Build history of the part. All positions in model axes, mm. A direction names the side the tool comes from. Coordinates: 2 decimals unless noted, no trailing zeros. Loops run counter-clockwise (first coordinate to the right, second up) from the corner with the lowest first, then second, coordinate; pieces in that order, holes last.
Item 1: Mould opens along Y. For faces 1 (the face through (2.321, 11.223, 1.479)), 2 (the face through (10, 0, 1)), 3 (the face through (5, 9, 1)) say: released by +Y, released by -Y, zero draft, split by the parting line, or undercut.
Item 2: Flat gauge pins, fed straight in: pin 1 (1.6 mm diameter, centred on x = 17.5, y = 2.5, fed in from -Z); pin 2 (1.5 mm diameter, centred on x = 11.5, z = 2.5, fed in from +Y). Where does each tip first touch, or does it go through?
Item 3: 3-axis set-ups, long thin cutter, end or side, ignore diameter. For faces 4 (the face through (0, 7, 1)), 5 (the face through (13, 5, 1)): which of +Z, -Z, +X, -X, +Y, -Y reach the whole face in a straight line?
Item 4: Cut at B-B (y = 9.86). List the corners of the cut face in (x, z) (3 decimals), and give its area (3 significant figures).
Item 5: Drill centre lines: line 1 along Y through (x, z) = (2.5, 1.9) (3 decimals); line 2 along Y through (x, z) = (17.5, 1.55) (3 decimals); line 3 along Y through (x, z) = (3, 0.8). Where is each one in solid material? Low to high.
Item 6: Cut at C-C (z = 2.75). List the corners of the cut face in (x, y) (3 decimals).
Item 7: Cut at A-A (y = 2.5). List the corners of the cut face in (x, z) (3 decimals).
from build123d import *

# Parameters (mm, degrees)
SKETCH1_R           = 1.375
BOSS_EXTRUDE1_DEPTH = 3


with BuildPart() as part:
    # Sketch1 → Boss-Extrude1 (new body)
    with BuildSketch(Plane.XY):
        Polygon((0, 0), (21, 0), (21, 5), (5, 5), (5, 13.36), (0, 13.36), align=None)
        with Locations((17.5, 2.5)):
            Circle(SKETCH1_R, mode=Mode.SUBTRACT)
        with Locations((2.5, 2.5)):
            Circle(SKETCH1_R, mode=Mode.SUBTRACT)
        with Locations((2.5, 9.86)):
            Circle(SKETCH1_R, mode=Mode.SUBTRACT)
    extrude(amount=BOSS_EXTRUDE1_DEPTH)


solid = part.part
Filled sheet:
1. face 1: undercut
1. face 2: released by -Y
1. face 3: zero draft
2. pin 1: passes through
2. pin 2: stops at y = 5
3. face 4: +Z, -Z, -X, +Y, -Y
3. face 5: +Z, -Z, +X, +Y
4. outline: (0, 0) - (1.125, 0) - (1.125, 3) - (0, 3) - close; (3.875, 0) - (5, 0) - (5, 3) - (3.875, 3) - close
4. area: 6.75 mm2
5. line 1: y = 0 to 1.125, 3.875 to 8.485, 11.235 to 13.36
5. line 2: y = 0 to 1.125, 3.875 to 5
5. line 3: y = 0 to 1.22, 3.78 to 8.58, 11.14 to 13.36
6. outline: (0, 0) - (21, 0) - (21, 5) - (5, 5) - (5, 13.36) - (0, 13.36) - close; hole circle Ø2.75 at (2.5, 2.5); hole circle Ø2.75 at (2.5, 9.86); hole circle Ø2.75 at (17.5, 2.5)
7. outline: (0, 0) - (1.125, 0) - (1.125, 3) - (0, 3) - close; (3.875, 0) - (16.125, 0) - (16.125, 3) - (3.875, 3) - close; (18.875, 0) - (21, 0) - (21, 3) - (18.875, 3) - close
